Model file for the job. Use its own axes, mm. A direction names the side the tool comes from. Coordinates: 2 decimals unless noted, no trailing zeros. Order: outer loops, then holes, each group sorted by start corner. A loop starts at its lowest first (then second) coordinate and runs counter-clockwise, first axis right, second up. Notation, with made-up numbers: M 45,64 L 78,64 A20 ccw 78,91 Z; hole C 2.5,17 d2. An arc over 180 degrees is marked long. Return JSON: item names as keys, results as strings.
```python
from build123d import *

# Parameters (mm, degrees)
F1_DEPTH       = 1200
F2_W           = 2
F2_H           = 430
F3_DEPTH       = 648
F4_R           = 200
F5_W           = 600
F5_H           = 460
F6_DEPTH       = 300
F7_W           = 596
F7_H           = 456
F8_DEPTH       = 300
F9_R           = 50
F10_R          = 50
F11_R          = 50
F12_R          = 12.5
F13_DEPTH      = 30
F14_W          = 30
F14_H          = 30
F15_DEPTH      = 865
F16_W          = 540
F16_H          = 30
F17_DEPTH      = 1110
F17_DEPTH_BACK = 30
F18_R          = 25
F19_DEPTH      = 2


with BuildPart() as f1:
    # F0 (on Right) → F1 (new body)
    with BuildSketch(Plane.YZ):
        Polygon((30, 0), (0, 0), (0, -30), (650, -30), (650, 400), (648, 400), (648, 0), (580, 0), (580, -28), (30, -28), align=None)
    extrude(amount=F1_DEPTH)

    # F2 (on Front) → F3 (join, through all)
    with BuildSketch(Plane.XZ):
        with Locations((1, 185)):
            Rectangle(F2_W, F2_H)
        with Locations((1199, 185)):
            Rectangle(F2_W, F2_H)
    extrude(amount=-F3_DEPTH)

    # F4
    f4_edges = [f1.edges().sort_by_distance(p)[0] for p in [
        (1, 0, 400),
        (1199, 0, 400),
    ]]
    fillet(f4_edges, radius=F4_R)

    # F5 (on face) → F6 (join)
    with BuildSketch(Plane(origin=(0, 0, -30), x_dir=(1, 0, 0), z_dir=(0, 0, -1))):
        with Locations((347, -305)):
            Rectangle(F5_W, F5_H)
    extrude(amount=F6_DEPTH)

    # F7 (on face) → F8 (cut)
    with BuildSketch(Plane.XY.offset(-28)):
        with Locations((347, 305)):
            Rectangle(F7_W, F7_H)
    extrude(amount=-F8_DEPTH, mode=Mode.SUBTRACT)

    # F9
    f9_edges = [f1.edges().sort_by_distance(p)[0] for p in [
        (645, 533, -178),
        (49, 533, -178),
        (49, 77, -178),
        (645, 77, -178),
    ]]
    fillet(f9_edges, radius=F9_R)

    # F10
    f10_edges = [f1.edges().sort_by_distance(p)[0] for p in [
        (47, 535, -180),
        (47, 75, -180),
        (647, 75, -180),
        (647, 535, -180),
    ]]
    fillet(f10_edges, radius=F10_R)

    # F11
    f11_edges = [f1.edges().sort_by_distance(p)[0] for p in [
        (347, 533, -328),
        (47, 305, -330),
    ]]
    fillet(f11_edges, radius=F11_R)

    # F12 (on face) → F13 (cut, through all)
    with BuildSketch(Plane.XY):
        with Locations((257, 614)):
            Circle(F12_R)
        with Locations((437, 614)):
            Circle(F12_R)
    extrude(amount=-F13_DEPTH, mode=Mode.SUBTRACT)

    # F14 (on face) → F15 (join)
    with BuildSketch(Plane(origin=(0, 0, -30), x_dir=(1, 0, 0), z_dir=(0, 0, -1))):
        with Locations((45, -45)):
            Rectangle(F14_W, F14_H)
        with Locations((1155, -45)):
            Rectangle(F14_W, F14_H)
        with Locations((1155, -555)):
            Rectangle(F14_W, F14_H)
        with Locations((45, -555)):
            Rectangle(F14_W, F14_H)
    extrude(amount=F15_DEPTH)

    # F16 (on face) → F17 (join, two sides)
    with BuildSketch(Plane.YZ.offset(60)) as f17_sk:
        with Locations((300, -760)):
            Rectangle(F16_W, F16_H)
    extrude(amount=F17_DEPTH)
    extrude(f17_sk.sketch, amount=-F17_DEPTH_BACK)

    # F18 (on face) → F19 (cut, through all)
    with BuildSketch(Plane.XY.offset(-328)):
        with Locations((347, 305)):
            Circle(F18_R)
    extrude(amount=-F19_DEPTH, mode=Mode.SUBTRACT)


solid = f1.part
```
Item 1: Saw through at D-D (z = -92). Count the separate pieces of the cut face and the enclosed holes in it, and give its area (3 significant figures).
Check result:
{"separate pieces": "5", "enclosed holes": "1", "area": "7,820 mm2"}
Item 2: Saw through at C-C (y = 263.5). Write the cut outline in (x, z).
Check result:
{"outline": "M 0,-30 L 47,-30 L 47,-280 A50 ccw 97,-330 L 597,-330 A50 ccw 647,-280 L 647,-30 L 1200,-30 L 1200,400 L 1198,400 L 1198,-28 L 645,-28 L 645,-278 A50 cw 595,-328 L 99,-328 A50 cw 49,-278 L 49,-28 L 2,-28 L 2,400 L 0,400 Z; M 30,-775 L 1170,-775 L 1170,-745 L 30,-745 Z"}
Item 3: 3-axis set-ups, long thin cutter, end or side, ignore diameter. For faces 5 (the flat face through (1155, 60, -382)), 6 (the flat face through (1140, 45, -382)), 7 (the flat face through (60, 555, -382)), 8 (the cylindrical face through (61.258, 90.036, -156.75)): which of +Z, -Z, +X, -X, +Y, -Y reach the whole face in a straight line?
Check result:
{"face 5": "+X, -X", "face 6": "+Y, -Y", "face 7": "+Y", "face 8": "-X"}
Item 4: Saw through at A-A (z = -691). Write the cut outline in (x, y).
Check result:
{"outline": "M 30,30 L 60,30 L 60,60 L 30,60 Z; M 30,540 L 60,540 L 60,570 L 30,570 Z; M 1140,30 L 1170,30 L 1170,60 L 1140,60 Z; M 1140,540 L 1170,540 L 1170,570 L 1140,570 Z"}
Item 5: Drop flat-ended pins along their axis: pin 1 Ø24 at (y, z) = (39.5, -372.5) entering from +X; pin 2 Ø24 at (y, z) = (548, -519.5) entering from -X; pin 3 Ø9 at (x, z) = (45, -428.5) entering from +Y. Give the stop position or say it passes through.
Check result:
{"pin 1": "stops at x = 1170", "pin 2": "stops at x = 30", "pin 3": "stops at y = 570"}
Item 6: Saw through at B-B (x = 1092). Write the cut outline in (y, z).
Check result:
{"outline": "M 0,-30 L 650,-30 L 650,400 L 648,400 L 648,0 L 580,0 L 580,-28 L 30,-28 L 30,0 L 0,0 Z; M 30,-775 L 570,-775 L 570,-745 L 30,-745 Z"}
Item 7: Wall check: line 1 (X direction, y = 614, z = -14.75); line 2 (Y direction, x = 437, z = -12.75); line 3 (Y direction, x = 515, z = -174). Give the ranges that are in metal, low to high.
Check result:
{"line 1": "x = 0 to 244.5, 269.5 to 424.5, 449.5 to 1200", "line 2": "y = 0 to 30, 580 to 601.5, 626.5 to 650", "line 3": "y = 75 to 77, 533 to 535"}
Item 8: Pull direction Y, two halves, no side cores. Call faces 1 (the flat face through (857, 309, -28)), 2 (the cylindrical face through (61.258, 519.964, -156.75)), 3 (the cylindrical face through (343.5, 520.742, -314.964)), 4 (the cylindrical face through (1199.014, 57.032, 339.858)): +Y half, -Y half, draft (parallel to the pull), parting line (faces both ways), or undercut.
Check result:
{"face 1": "undercut", "face 2": "undercut", "face 3": "+Y half", "face 4": "-Y half"}
